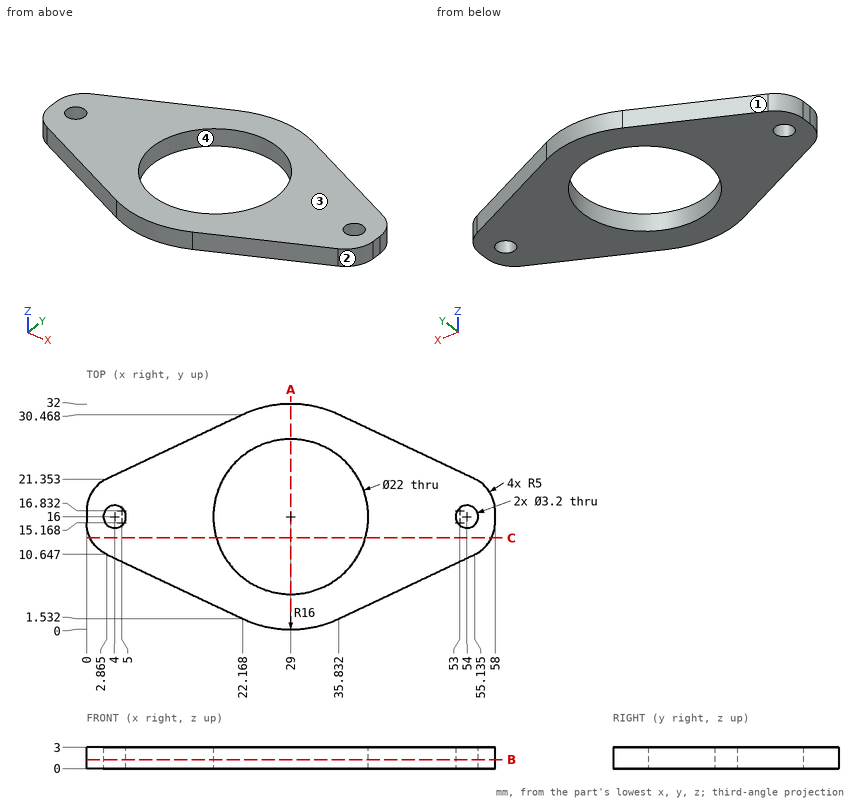
Source: three-view drawing plus pictorial views. Frame: mm from the lowest corner of the part. Give positions to 0.01 mm unless a question says otherwise; leave off trailing zeros. Order: outer loops, then holes, each group sorted by start corner. A loop starts at its lowest first (then second) coordinate and runs counter-clockwise, first axis right, second up. Notation, with made-up numbers: (7.25, 12) -> (36.25, 12) arc R17 ccw to (36.25, 24) -> close; hole circle Ø4 at (-13.5, -2). An arc over 180 degrees is marked (long way). Use a Markdown table: item, result.
Q1. Section B-B (z = 1.25). Return the cut outline in (x, y) (1 decimal), and give its area (3 significant figures).
A:
| item | result |
|---|---|
| outline | (0, 15.2) arc R5 ccw to (2.9, 10.6) -> (22.2, 1.5) arc R16 ccw to (35.8, 1.5) -> (55.1, 10.6) arc R5 ccw to (58, 15.2) -> (58, 16.8) arc R5 ccw to (55.1, 21.4) -> (35.8, 30.5) arc R16 ccw to (22.2, 30.5) -> (2.9, 21.4) arc R5 ccw to (0, 16.8) -> close; hole circle Ø3.2 at (4, 16); hole circle Ø22 at (29, 16); hole circle Ø3.2 at (54, 16) |
| area | 839 mm^2 |
Q2. Section C-C (y = 13). Return the cut outline in (x, z) (1 decimal).
A:
| item | result |
|---|---|
| outline | (0.5, 0) -> (18.4, 0) -> (18.4, 3) -> (0.5, 3) -> close; (39.6, 0) -> (57.5, 0) -> (57.5, 3) -> (39.6, 3) -> close |
Q3. Section A-A (x = 29). Return the cut outline in (y, z).
A:
| item | result |
|---|---|
| outline | (0, 0) -> (5, 0) -> (5, 3) -> (0, 3) -> close; (27, 0) -> (32, 0) -> (32, 3) -> (27, 3) -> close |
Q4. First-contact query: P1, Ø1.5, axis at x = 44, z = 1.5, coming from the +Y side (1 decimal). Flat tip, straight axial feed; report the tip coordinate or a pass-through.
A:
| item | result |
|---|---|
| P1 | y = 27 |
Q5. Material intervals for line 1 (X direction, y = 16.5, z = 2.5); line 2 (X direction, y = 8, z = 2.6); line 3 (Y direction, x = 4, z = 1.8), sorted ascending. Write a range as [from, to].
A:
| item | result |
|---|---|
| line 1 | [0, 2.48], [5.52, 18.01], [39.99, 52.48], [55.52, 58] |
| line 2 | [8.47, 21.45], [36.55, 49.53] |
| line 3 | [10.11, 14.4], [17.6, 21.89] |
Q6. Pull-direction query (X, two-part tool) for the marked faces 1, 2, 3 and 4; classes: +X half, -X half, draft (parallel to the pull), parting line (faces both ways), or undercut.
A:
| item | result |
|---|---|
| face 1 | -X half |
| face 2 | +X half |
| face 3 | draft |
| face 4 | undercut |
